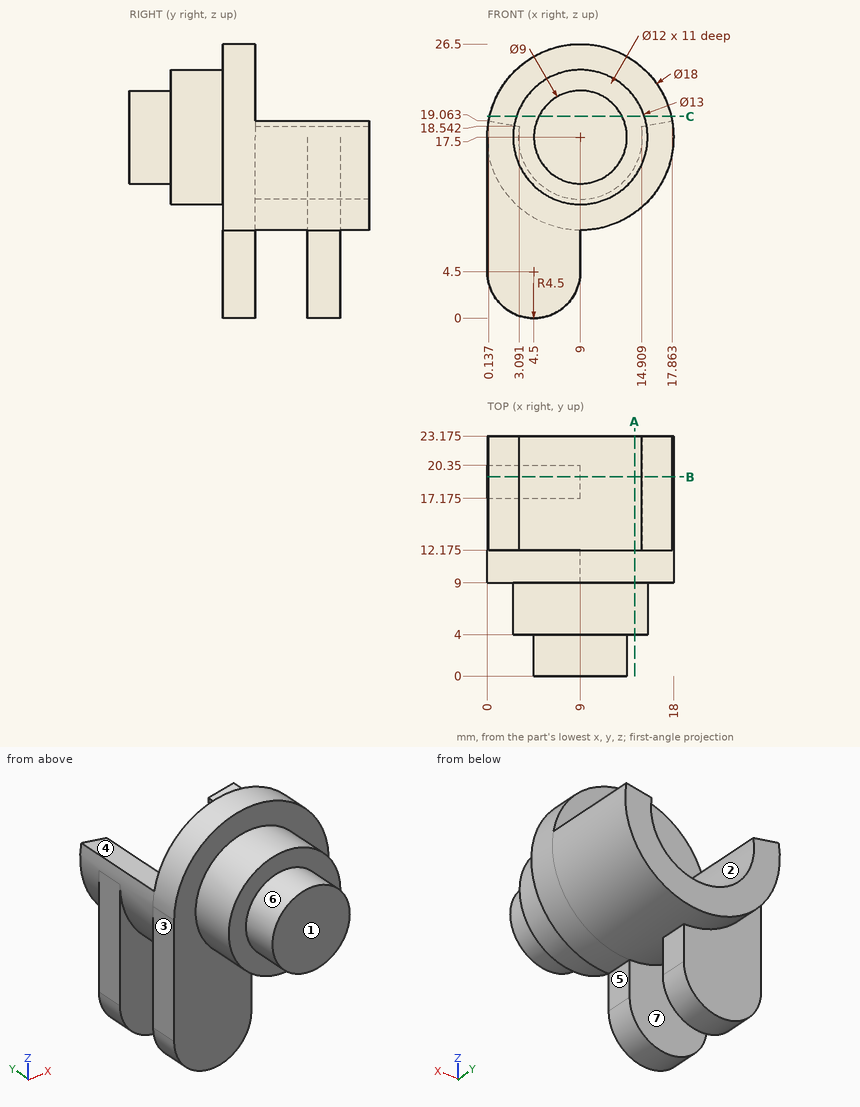
The figure shows three views and two pictorial views of one solid part (mm, origin at its lowest corner). Answer the questions. A direction names the side the tool comes from. Give positions to 0.01 mm unless a question says otherwise; leave off trailing zeros. Loops run counter-clockwise (first coordinate to the right, second up) from the corner with the lowest first, then second, coordinate; pieces in that order, holes last. Notation, with made-up numbers: (-4, 26) -> (32, 26) arc R15 cw to (32, 49) -> close; hole circle Ø3 at (77.25, 45.25). An arc over 180 degrees is marked (long way). Use a Markdown table: item, result. Add a question column.
1. Determine the mould class of the marked faces 1, 2 and 3 for opening direction X: released by +X, released by -X, zero draft, split by the parting line, or undercut.
2. Section A-A on x = 14.25 is taken. Determine the outline of the cut face in (y, z) (1 decimal), and give its area (3 significant figures).
3. Find the intervals of material crossed by probe 1 along X at (y, z) = (15.5, 17.5); probe 2 along Z at (x, y) = (9, 16); probe 3 along X at (y, z) = (16.25, 12.75) (1 decimal), in increasing order.
4. Section B-B on y = 19.25 is taken. Determine the outline of the cut face in (x, z).
5. Flat-ended cylindrical pins translate along their axes: pin 1 Ø8 at (x, z) = (11.5, 9) entering from -Y; pin 2 Ø1 at (y, z) = (10.5, 6.5) entering from +X; pin 3 Ø1.5 at (y, z) = (10.5, 10.5) entering from +X (1 decimal). Find the tip coordinate at first contact, or state that the pin passes through.
6. Section C-C on z = 19.5 is taken. Determine the outline of the cut face in (x, y) (1 decimal), and give its area (3 significant figures).
7. For the marked faces 4, 5, 6 and 7, determine the directions among +Z, -Z, +X, -X, +Y, -Y from which every point of the face is accessible in a straight line to the end or side of a thin tool.
Results below:
| question | item | result |
|---|---|---|
| 1 | face 1 | zero draft |
| 1 | face 2 | undercut |
| 1 | face 3 | released by -X |
| 2 | outline | (4, 13.7) -> (9, 13.7) -> (9, 10.2) -> (23.2, 10.2) -> (23.2, 14.6) -> (12.2, 14.6) -> (12.2, 24.8) -> (9, 24.8) -> (9, 21.3) -> (4, 21.3) -> close |
| 2 | area | 133 mm^2 |
| 3 | probe 1 | x = 0 to 3, 15 to 18 |
| 3 | probe 2 | z = 8.5 to 11.5 |
| 3 | probe 3 | x = 1.4 to 5.3, 12.7 to 16.6 |
| 4 | outline | (0, 4.5) arc R4.5 ccw to (9, 4.5) -> (9, 8.5) arc R9 ccw to (17.86, 19.06) -> (14.91, 18.54) arc R6 cw (long way) to (3.09, 18.54) -> (0.14, 19.06) arc R9 ccw to (0, 17.5) -> close |
| 5 | pin 1 | stops at y = 4 |
| 5 | pin 2 | stops at x = 9 |
| 5 | pin 3 | stops at x = 15.5 |
| 6 | outline | (0.2, 9) -> (2.8, 9) -> (2.8, 4) -> (5, 4) -> (5, 0) -> (13, 0) -> (13, 4) -> (15.2, 4) -> (15.2, 9) -> (17.8, 9) -> (17.8, 12.2) -> (0.2, 12.2) -> close |
| 6 | area | 150 mm^2 |
| 7 | face 4 | +Z, +Y |
| 7 | face 5 | -Z, +X, +Y, -Y |
| 7 | face 6 | -Y |
| 7 | face 7 | -Z, -X |
